```python
from build123d import *

# Parameters (mm, degrees)
SKETCH1_W           = 15
SKETCH1_H           = 8
BOSS_EXTRUDE1_DEPTH = 10
SKETCH2_W           = 15
SKETCH2_H           = 2
CUT_EXTRUDE1_DEPTH  = 7
FILLET1_R           = 0.6


with BuildPart() as part:
    # Sketch1 → Boss-Extrude1 (new body)
    with BuildSketch(Plane.XY):
        with Locations((-7.5, 4)):
            Rectangle(SKETCH1_W, SKETCH1_H)
    extrude(amount=BOSS_EXTRUDE1_DEPTH)

    # Sketch2 → Cut-Extrude1 (cut)
    with BuildSketch(Plane.XY.offset(10)):
        with Locations((-7.5, 4)):
            Rectangle(SKETCH2_W, SKETCH2_H)
    extrude(amount=-CUT_EXTRUDE1_DEPTH, mode=Mode.SUBTRACT)

    # Fillet1
    fillet1_edges = [part.edges().sort_by_distance(p)[0] for p in [
        (-15, 6.5, 10),
        (0, 6.5, 10),
        (-15, 1.5, 10),
        (-7.5, 0, 10),
        (-15, 4, 3),
        (-15, 3, 6.5),
        (-15, 5, 6.5),
        (0, 4, 3),
        (0, 5, 6.5),
        (0, 3, 6.5),
        (-7.5, 3, 10),
        (-7.5, 5, 10),
        (0, 1.5, 10),
        (-7.5, 0, 0),
        (-15, 4, 0),
        (-7.5, 8, 0),
        (0, 4, 0),
        (0, 0, 5),
        (-15, 0, 5),
        (-15, 8, 5),
        (0, 8, 5),
        (-7.5, 8, 10),
    ]]
    fillet(fillet1_edges, radius=FILLET1_R)


solid = part.part
```
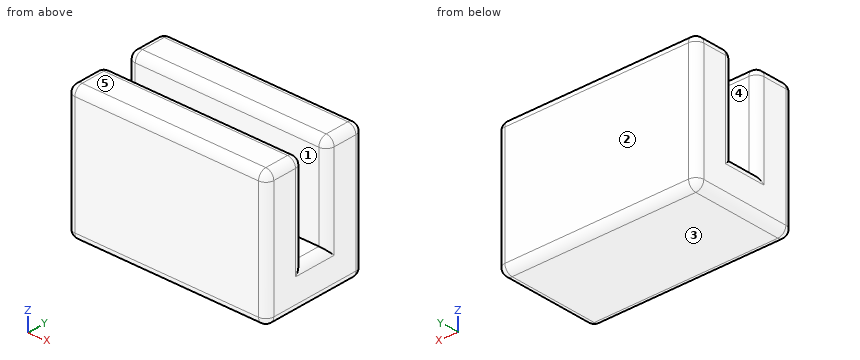
CAD build for the part. Positions are in the model's coordinates, mm. Face numbers are marked on the shaded views. A direction names the side the tool comes from. Round coordinates to 2 decimals unless told otherwise and drop trailing zeros. Loops run counter-clockwise (first coordinate to the right, second up) from the corner with the lowest first, then second, coordinate; pieces in that order, holes last. Notation, with made-up numbers: (86, 3.25) - (131, 3.25) arc R17 cw to (131, 21.25) - close; hole circle Ø6 at (-30, 29.25). An arc over 180 degrees is marked (long way). Return JSON: item names as keys, results as strings. Group by question number.
Q1. Band-saw the part on A-A on z = 4.75. Give the cut face in (x, y).
Q2. Two-plate mould, pull along Z, no slides. Class the marked faces 3, 4 and 5: +Z half, -Z half, draft (parallel to the pull), parting line (faces both ways), or undercut.
Q3. Band-saw the part on B-B on y = 3.25. Give the cut face in (x, z).
Q4. Flat gauge pin, fed straight in: pin 1 Ø1.6 at (x, y) = (-7, 4) entering from +Z. Where does the tip first touch, or does it go through?
Q5. Tool access for the marked faces 1 and 2: list every direction of +Z, -Z, +X, -X, +Y, -Y with a clear straight run to the whole face (end or side of a thin tool).
Q6. Drill centre lines: line 1 along Y through (x, z) = (-13, 5.25); line 2 along Z through (x, y) = (-8.75, 0.5); line 3 along Y through (x, z) = (-10.75, 0.5). Where is each one in solid material? Low to high. Write a range as [from, to].
Q7. Band-saw the part on C-C on x = -4.75. Give the cut face in (y, z).
Solutions:
{
 "1": {"outline": "(-15, 0.6) arc R0.6 ccw to (-14.4, 0) - (-0.6, 0) arc R0.6 ccw to (0, 0.6) - (0, 2.4) arc R0.6 ccw to (-0.6, 3) - (-14.4, 3) arc R0.6 ccw to (-15, 2.4) - close; (-15, 5.6) arc R0.6 ccw to (-14.4, 5) - (-0.6, 5) arc R0.6 ccw to (0, 5.6) - (0, 7.4) arc R0.6 ccw to (-0.6, 8) - (-14.4, 8) arc R0.6 ccw to (-15, 7.4) - close"},
 "2": {"face 3": "-Z half", "face 4": "draft", "face 5": "+Z half"},
 "3": {"outline": "(-15, 0.6) arc R0.6 ccw to (-14.4, 0) - (-0.6, 0) arc R0.6 ccw to (0, 0.6) - (0, 2.4) arc R0.6 ccw to (-0.6, 3) - (-14.4, 3) arc R0.6 ccw to (-15, 2.4) - close"},
 "4": {"pin 1": "stops at z = 3"},
 "5": {"face 1": "+Z, +X, -X", "face 2": "+Z, -Z, +X, -X, +Y"},
 "6": {"line 1": "y = [0, 3], [5, 8]", "line 2": "z = [0.01, 9.99]", "line 3": "y = [0.01, 7.99]"},
 "7": {"outline": "(0, 0.6) arc R0.6 ccw to (0.6, 0) - (7.4, 0) arc R0.6 ccw to (8, 0.6) - (8, 9.4) arc R0.6 ccw to (7.4, 10) - (5.6, 10) arc R0.6 ccw to (5, 9.4) - (5, 3) - (3, 3) - (3, 9.4) arc R0.6 ccw to (2.4, 10) - (0.6, 10) arc R0.6 ccw to (0, 9.4) - close"}
}
